```python
from build123d import *

# Parameters (mm, degrees)
SKETCH1_W = 1.525
SKETCH1_H = 5.6
FILLET1_R = 0.25


with BuildPart() as part:
    # Sketch1 → Revolve1 (revolve)
    with BuildSketch(Plane.XY, mode=Mode.PRIVATE) as revolve1_sk:
        with Locations((0.7625, 2.8)):
            Rectangle(SKETCH1_W, SKETCH1_H)
        Polygon((0, 5.6), (1.525, 5.6), (1.31, 5.972390924), (1.31, 6.352390924), (2.86, 6.352390924), (2.86, 7.942390924), (0, 7.942390924), align=None)
    revolve(revolve1_sk.sketch.rotate(Axis((-6, 0, 0), (0, 1, 0)), 90), axis=Axis((-6, 0, 0), (0, 1, 0)))

    # Fillet1
    fillet1_edges = [part.edges().sort_by_distance(p)[0] for p in [
        (-6, 6.352390924, 7.31),
    ]]
    fillet(fillet1_edges, radius=FILLET1_R)


solid = part.part
```
CAD build for the part. Positions are in the model's coordinates, mm. Give positions to 0.01 mm unless a question says otherwise; leave off trailing zeros. Write each loop counter-clockwise with the first axis right and the second up, starting at its lowest first coordinate (ties: lowest second). Pieces come first, ordered by that corner, then holes. Notation, with made-up numbers: (48.25, 13.5) -> (93.25, 13.5) arc R20 cw to (93.25, 42.5) -> close; hole circle Ø7 at (41, 4). An arc over 180 degrees is marked (long way). Write each question's results on one line, items separated by ' | '.
1. Cut at D-D, the plane y = 7.5. Write the cut outline in (x, z).
Geometry check:
outline: circle Ø17.72 at (-6, 0); hole circle Ø12 at (-6, 0)
2. Two-plate mould, pull along Z, no slides. Class faces 1 (the cylindrical face through (-13.46, 2.84, 0.98)), 2 (the cylindrical face through (-7.802, 3.916, -5.723)), 3 (the flat face through (-10, 6.352, 7)): pulls with the +Z half, pulls with the -Z half, needs draft (parallel to the pull), parting line crosses it, or undercut.
Geometry check:
face 1: parting line crosses it | face 2: undercut | face 3: needs draft
3. Wall check: probe 1 along X at (y, z) = (2.25, 0) (3 decimals); probe 2 along X at (y, z) = (2.5, 1); probe 3 along Z at (x, y) = (-9.25, 4). Give the ranges that are in metal, low to high. Write a range as [from, to].
Geometry check:
probe 1: [-13.525, -12], [0, 1.525] | probe 2: [-13.46, -11.92], [-0.08, 1.46] | probe 3: [-6.79, -5.04], [5.04, 6.79]
4. Cut at B-B, the plane x = -6. Write the cut outline in (y, z) (3 decimals).
Geometry check:
outline: (0, -7.525) -> (5.6, -7.525) -> (5.972, -7.31) -> (6.102, -7.31) arc R0.25 cw to (6.352, -7.56) -> (6.352, -8.86) -> (7.942, -8.86) -> (7.942, -6) -> (0, -6) -> close; (0, 6) -> (7.942, 6) -> (7.942, 8.86) -> (6.352, 8.86) -> (6.352, 7.56) arc R0.25 cw to (6.102, 7.31) -> (5.972, 7.31) -> (5.6, 7.525) -> (0, 7.525) -> close
5. Cut at A-A, the plane z = 0. Write the cut outline in (x, y) (3 decimals), then the cut area to 3 significant figures.
Geometry check:
outline: (-14.86, 6.352) -> (-13.56, 6.352) arc R0.25 cw to (-13.31, 6.102) -> (-13.31, 5.972) -> (-13.525, 5.6) -> (-13.525, 0) -> (-12, 0) -> (-12, 7.942) -> (-14.86, 7.942) -> close; (0, 0) -> (1.525, 0) -> (1.525, 5.6) -> (1.31, 5.972) -> (1.31, 6.102) arc R0.25 cw to (1.56, 6.352) -> (2.86, 6.352) -> (2.86, 7.942) -> (0, 7.942) -> close | area: 28.3 mm²
6. Drop flat-ended pins along their axis: P1, Ø1, axis at x = -7.5, y = 4, coming from the -Z side; P2, Ø2, axis at y = 5.5, z = 2.5, coming from the -X side; P3, Ø3, axis at y = 3.5, z = 4.5, coming from the -X side. Give the stop position or say it passes through.
Geometry check:
P1: z = -7.46 | P2: x = -14.64 | P3: x = -12.9
7. Cut at C-C, the plane y = 5.25. Write the cut outline in (x, z) (3 decimals), then the cut area to 3 significant figures.
Geometry check:
outline: circle Ø15.05 at (-6, 0); hole circle Ø12 at (-6, 0) | area: 64.8 mm²
